Check sheet for the modelled part. Datum: model origin and axes. Units: mm. A direction names the side the tool comes from. Coordinates: 2 decimals unless noted, no trailing zeros. Loops run counter-clockwise (first coordinate to the right, second up) from the corner with the lowest first, then second, coordinate; pieces in that order, holes last.
```python
from build123d import *
from build123d import SkipClean  # not in build123d's __all__

# Parameters (mm, degrees)
F1_DEPTH       = 19.88
F2_R           = 4.382
F3_R           = 3.81
F4_DEPTH       = 2.5
F4_DEPTH_BACK  = 5
F5_R           = 2.2987
F6_DEPTH       = 2.501
F7_R           = 4.01
F8_DEPTH       = 3
F9_R           = 1.8288
F10_DEPTH      = 19.8810001
F11_R          = 2.53
F12_DEPTH      = 21.176
F14_W          = 12.0765847373
F14_H          = 13.03
F15_DEPTH      = 11.351
F16_W          = 10.5
F16_H          = 3.36
F17_DEPTH      = 11.351
F18_R          = 2.865
F19_DEPTH      = 20
F19_DEPTH_BACK = 0.5
F20_R          = 2.865
F21_DEPTH      = 20.001


# Not quite as in the source:
# - after a boolean that leaves OpenCascade's solid faulty, fix() repairs it


with BuildPart() as f1:
    # F0 (on Top) → F1 (new body)
    with BuildSketch(Plane.XY):
        with BuildLine():
            Line((0, -11.375), (0, -26.185))
            Line((0, -26.185), (29.875, -26.185))
            Line((29.875, -26.185), (29.875, -21.185))
            Line((29.875, -21.185), (21.175, -21.185))
            Line((21.175, -21.185), (21.175, 17.015))
            Line((21.175, 17.015), (16.7292900036, 21.065))
            Line((16.7292900036, 21.065), (11.8792900036, 21.065))
            Line((11.8792900036, 21.065), (9.825, 15.6823642592))
            Line((9.825, 15.6823642592), (9.825, 5.7323642592))
            ThreePointArc((9.825, 5.7323642592), (9.8639816618, -5.6650234577), (0, -11.375))
        make_face()
    extrude(amount=F1_DEPTH)

    # F2
    f2_edges = [f1.edges().sort_by_distance(p)[0] for p in [
        (21.175, -21.185, 9.94),
    ]]
    fillet(f2_edges, radius=F2_R)

    # F3 (on face) → F4 (cut, two sides)
    with BuildSketch(Plane(origin=(0, -21.185, 0), x_dir=(-1, 0, 0), z_dir=(0, 1, 0))) as f4_sk:
        with Locations((-25.557, 9.94)):
            Circle(F3_R)
    extrude(amount=-F4_DEPTH, mode=Mode.SUBTRACT)
    extrude(f4_sk.sketch, amount=F4_DEPTH_BACK, mode=Mode.SUBTRACT)

    # F5 (on face) → F6 (cut, through all)
    with BuildSketch(Plane(origin=(0, -23.685, 0), x_dir=(-1, 0, 0), z_dir=(0, 1, 0))):
        with Locations((-25.557, 9.94)):
            Circle(F5_R)
    extrude(amount=-F6_DEPTH, mode=Mode.SUBTRACT)

    # F7 (on face) → F8 (cut)
    with BuildSketch(Plane.XY.offset(19.88)):
        with Locations((15.475, -15.525)):
            Circle(F7_R)
        with Locations((0, -14.955)):
            Circle(F7_R)
        with Locations((14.915, 0)):
            Circle(F7_R)
    extrude(amount=-F8_DEPTH, mode=Mode.SUBTRACT)

    # F9 (on face) → F10 (cut, through all)
    with BuildSketch(Plane.XY.offset(19.88)):
        with Locations((14.915, 0)):
            Circle(F9_R)
        with Locations((15.475, -15.525)):
            Circle(F9_R)
        with Locations((0, -14.955)):
            Circle(F9_R)
    extrude(amount=-F10_DEPTH, mode=Mode.SUBTRACT)

    # F11 (on face) → F12 (cut, through all)
    with BuildSketch(Plane.YZ.offset(21.175)):
        with Locations((6.145, 9.89)):
            Circle(F11_R)
    extrude(amount=-F12_DEPTH, mode=Mode.SUBTRACT)

    # F13: F1 across plane


with BuildPart() as f1_1:
    add(f1.part, clean=False)
    with SkipClean():  # cleaning this boolean's faces spoils the solid; the shape is the same uncleaned
        add(f1.part.mirror(Plane.YZ), clean=False)

    # F14 (on face) → F15 (cut, through all)
    with BuildSketch(Plane.YZ.offset(21.175)):
        with Locations((15.9632923686, 9.94)):
            Rectangle(F14_W, F14_H)
    extrude(amount=-F15_DEPTH, mode=Mode.SUBTRACT)

    add(f1_1.part.fix(), mode=Mode.REPLACE)

    # F16 (on face) → F17 (cut, through all)
    with BuildSketch(Plane(origin=(-21.175, 0, 0), x_dir=(0, -1, 0), z_dir=(-1, 0, 0))):
        with Locations((-16.215, 9.94)):
            Rectangle(F16_W, F16_H)
    extrude(amount=-F17_DEPTH, mode=Mode.SUBTRACT)

    # F18 (on face) → F19 (join, two sides)
    with BuildSketch(Plane.XY.offset(19.88)) as f19_sk:
        with Locations((15.875, 15.17)):
            Circle(F18_R)
    extrude(amount=-F19_DEPTH)
    extrude(f19_sk.sketch, amount=F19_DEPTH_BACK)

    # F20 (on face) → F21 (cut, through all)
    with BuildSketch(Plane.XY.offset(19.88)):
        with Locations((-15.875, 15.17)):
            Circle(F20_R)
    extrude(amount=-F21_DEPTH, mode=Mode.SUBTRACT)


solid = f1_1.part
```
1) Section check B-B on y = -6. Enter the section's corners in (x, z) (3 decimals).
Answer sheet:
outline: (-21.175, 0) - (-9.664, 0) - (-9.664, 19.88) - (-21.175, 19.88) - close; (9.664, 0) - (21.175, 0) - (21.175, 19.88) - (9.664, 19.88) - close
2) Set-up check for faces 1 (the flat face through (-10.867, 18.411, 4.072)), 2 (the flat face through (16, 9.925, 10)), 3 (the cylindrical face through (-21.92, -21.82, 11.08)), 4 (the flat face through (13, 14, 3.425)), 5 (the flat face through (-15.6, 18.3, 11.62)): record each of +Z, -Z, +X, -X, +Y, -Y from which the full face is reachable in a straight line by a thin tool's end or side.
Answer sheet:
face 1: +Z, -Z, +Y
face 2: +X
face 3: +Y
face 4: none
face 5: -X, +Y
3) Depth check by flat-ended pin: pin 1 (6.5 mm diameter, centred on x = -15.5, y = -17, fed in from +Z); pin 2 (3.5 mm diameter, centred on x = -15.875, y = 15.17, fed in from +Z); pin 3 (3 mm diameter, centred on y = -8, z = 2, fed in from -X) (3 decimals); pin 4 (1.5 mm diameter, centred on y = -9.5, z = 11, fed in from +X) (3 decimals). Enter the tip coordinate at first touch or a pass-through.
Answer sheet:
pin 1: stops at z = 19.88
pin 2: passes through
pin 3: stops at x = -21.175
pin 4: stops at x = 21.175
4) Scan lines: line 1 (Y direction, x = 0, z = 4.25) (3 decimals); line 2 (Y direction, x = 19, z = 10) (3 decimals); line 3 (X direction, y = -14, z = 12.5) (3 decimals). Record each from-to range of solid material in increasing order.
Answer sheet:
line 1: y = -26.185 to -16.784, -13.126 to -11.375
line 2: y = -26.185 to 3.617, 8.673 to 9.925
line 3: x = -21.175 to -16.484, -14.466 to -1.56, 1.56 to 14.466, 16.484 to 21.175
5) Section check C-C on z = 9.25. Give the number of separate pieces and of enclosed holes in the cut face, plus the area to 3 significant figures.
Answer sheet:
separate pieces: 6
enclosed holes: 5
area: 1,030 mm2
6) Mould release check, pull along X, two halves, no side actions. Record for faces 6 (the cylindrical face through (-15.58, 8.56, 10.65)), 7 (the flat face through (-14.5, -17.3, 16.88)), 8 (the flat face through (21.175, -4, 10)): +X half, -X half, draft (parallel to the pull), parting line (faces both ways), or undercut.
Answer sheet:
face 6: draft
face 7: undercut
face 8: +X half
7) Section check D-D on x = 7. Enter the section's corners in (y, z) (3 decimals).
Answer sheet:
outline: (-26.185, 0) - (-8.966, 0) - (-8.966, 19.88) - (-26.185, 19.88) - close
8) Section check A-A on y = 0. Enter the section's corners in (x, z) (3 decimals), plus the area to 3 significant figures.
Answer sheet:
outline: (-21.175, 0) - (-16.744, 0) - (-16.744, 16.88) - (-18.925, 16.88) - (-18.925, 19.88) - (-21.175, 19.88) - close; (-13.086, 0) - (-11.375, 0) - (-11.375, 16.88) - (-13.086, 16.88) - close; (11.375, 0) - (13.086, 0) - (13.086, 16.88) - (11.375, 16.88) - close; (16.744, 0) - (21.175, 0) - (21.175, 19.88) - (18.925, 19.88) - (18.925, 16.88) - (16.744, 16.88) - close
area: 221 mm2
